Here's how the part is built. I have some questions about the finished solid (model axes, mm). A direction names the side the tool comes from. Round coordinates to 2 decimals unless told otherwise and drop trailing zeros. Loops run counter-clockwise (first coordinate to the right, second up) from the corner with the lowest first, then second, coordinate; pieces in that order, holes last. Notation, with made-up numbers: (35.5, 80) -> (91.5, 80) arc R19 ccw to (91.5, 98) -> close; hole circle Ø8 at (71.25, 54). An arc over 180 degrees is marked (long way). Use one line per item in the form item = value. Start each with the question number.
Item 1: If we section it at C-C (x = 14): Write out the boundary of the cut face in (y, z), then the cut area to 3 significant figures.
Item 2: If I drill on L1, parallel to Y at x = 0.5, z = 3.75 (3 decimals); L2, parallel to X at y = 0, z = 6 (3 decimals); L3, parallel to Y at x = -2, z = 1.25, over which ranges is the centre line in solid material (lowest first)? Write a range as [from, to].
Item 3: For faces 4 (the face through (12.92, -21.56, 4.93)), 5 (the face through (2.865, 20.849, 5.07)), 6 (the face through (-2.15, 18, 5)), 7 (the face through (-3.15, 19, 5)), which set-ups out of +Z, -Z, +X, -X, +Y, -Y let a thin tool reach every point of the face, with its end or its side?
Item 4: Thinking about a two-plate mould opening in X: for faces 1 (the face through (15.558, 3.798, 4.93)), 2 (the face through (-2.15, -23, 5)), 3 (the face through (-10.68, -12.86, 5.07)), which applies, released by +X, released by -X, zero draft, split by the parting line, or undercut?
Item 5: If we section it at D-D (y = 9): Write out the boundary of the cut face in (x, z).
Item 6: I'm going to push flat-ended pins straight in: pin 1 Ø1 at (y, z) = (-11.5, 5) entering from -X; pin 2 Ø1.6 at (y, z) = (19, 6.5) entering from -X; pin 3 Ø1.6 at (y, z) = (-24, 5.5) entering from +X. Where does each tip first touch, or does it pass through?
Item 7: If we section it at A-A (y = 0): Write out the boundary of the cut face in (x, z) (3 decimals), then the cut area to 3 significant figures.
Item 8: If we section it at B-B (x = 0): Write out the boundary of the cut face in (y, z) (3 decimals), then the cut area to 4 significant figures.
Autodesk Inventor part; units mm, degrees
ref_plane "YZ Plane" through (0, 0, 0) normal (1, 0, 0) x (0, 1, 0)
ref_plane "XZ Plane" through (0, 0, 0) normal (0, 1, 0) x (-1, 0, 0)
ref_plane "XY Plane" through (0, 0, 0) normal (0, 0, 1) x (1, 0, 0)
sketch "Sketch1" plane through (0, 0, 0) normal (0, 0, 1) x (1, 0, 0)
  circle A0 centre (0, 0) radius 15.015
  circle A1 centre (0, 0) radius 16.015
  line L0 (-10, -12.5092) -> (-15, -28)
  line L1 (-15, -28) -> (15, -28)
  line L2 (15, -28) -> (10, -12.5092)
  line L3 (8.2846, -13.7057) -> (11.9301, -25)
  line L4 (11.9301, -25) -> (3.15, -25)
  line L5 (-11.9301, -25) -> (-8.2846, -13.7057)
  line L6 (-1.5, -14.9399) -> (-1.5, -14.515)
  line L7 (-1, -14.015) -> (1, -14.015)
  line L8 (1.5, -14.515) -> (1.5, -14.9399)
  arc A2 (-1, -14.015) -> (-1.5, -14.515) centre (-1, -14.515) ccw
  arc A3 (1.5, -14.515) -> (1, -14.015) centre (1, -14.515) ccw
  line L9 (2, -25) -> (2, -22) construction
  line L10 (2, -22) -> (-2, -22) construction
  line L11 (-2, -22) -> (-2, -25) construction
  line L12 (-2.15, -25) -> (-2.15, -21.85)
  line L13 (-2.15, -21.85) -> (2.15, -21.85)
  line L14 (2.15, -21.85) -> (2.15, -25)
  line L15 (-3.15, -25) -> (-3.15, -20.85)
  line L16 (-3.15, -20.85) -> (3.15, -20.85)
  line L17 (3.15, -20.85) -> (3.15, -25)
  line L18 (3.15, -25) -> (2.15, -25)
  line L19 (2.15, -25) -> (-2.15, -25)
  line L20 (-2.15, -25) -> (-3.15, -25)
  line L21 (-3.15, -25) -> (-11.9301, -25)
  line L22 (2, 20) -> (-2, 20) construction
  line L23 (-2, 20) -> (-2, 17) construction
  line L24 (-2, 17) -> (2, 17) construction
  line L25 (2, 17) -> (2, 20) construction
  line L26 (-2.15, 16.85) -> (-2.15, 20.15)
  line L27 (-2.15, 20.15) -> (2.15, 20.15)
  line L28 (2.15, 20.15) -> (2.15, 16.85)
  line L29 (2.15, 16.85) -> (-2.15, 16.85)
  line L30 (3.15, 15.7022) -> (3.15, 21.15)
  line L31 (3.15, 21.15) -> (-3.15, 21.15)
  line L32 (-3.15, 21.15) -> (-3.15, 15.7022)
  point P0 (0, -28)
  point P1 (-1.5, -14.015)
  point P2 (1.5, -14.015)
  point P3 (0, -14.015)
  point P4 (0, -15.015)
  point P5 (0, -22)
  point P6 (0, -25)
  point P7 (0, -25)
  point P8 (0, 17)
  dimension "d0" = 28
  dimension "d1" = 1
  dimension "d2" = 30
  dimension "d3" = 30.03
  dimension "d4" = 20
  dimension "d5" = 3
  dimension "d6" = 2
  dimension "d10" = 3
  dimension "d12" = 1
  dimension "d13" = 0.5
  dimension "d14" = 3
  dimension "d15" = 4
  dimension "d16" = 0.15
  dimension "d17" = 1
  dimension "d21" = 4
  dimension "d22" = 3
  dimension "d23" = 17
  dimension "d24" = 0.15
  dimension "d25" = 1
  dimension "d26" = 1
  dimension "d27" = 1
extrude "Extrusion1" add sketch "Sketch1" along normal blind 10 contours L6 A2 L7 A3 L8 A0 | A1 | A1 L32 L31 L30 | L2 L1 L0 A1 L5 L21 L20 L19 L18 L4 L3 | L18 L14 L13 L12 L20 L15 L16 L17 picked at (0.1669, -14.3455)
fillet "Fillet1" radius 4 6 edges at (10, -12.5092, 5) (8.2846, -13.7057, 5) (-8.2846, -13.7057, 5) (-10, -12.5092, 5) (3.15, 15.7022, 5) (-3.15, 15.7022, 5)
fillet "Fillet1" radius 2 4 edges at (11.9301, -25, 5) (-11.9301, -25, 5) (-3.15, -25, 5) (3.15, -25, 5)
fillet "Fillet1" radius 1 4 edges at (3.15, -20.85, 5) (-3.15, -20.85, 5) (3.15, 21.15, 5) (-3.15, 21.15, 5)
properties part number "Motor Reversed Mount Midsection" material "ABS Plastic"
Values found:
q1.outline = (-28, 0) -> (-24.9, 0) -> (-24.9, 10) -> (-28, 10) -> close; (-7.78, 0) -> (-5.43, 0) -> (-5.43, 10) -> (-7.78, 10) -> close; (5.43, 0) -> (7.78, 0) -> (7.78, 10) -> (5.43, 10) -> close
q1.area = 78.0 mm2
q2.L1 = [-28, -25], [-21.85, -20.85], [-16.007, -14.015], [15.007, 16.85], [20.15, 21.15]
q2.L2 = [-16.015, -15.015], [15.015, 16.015]
q2.L3 = [-28, -25], [-21.85, -20.85], [-15.89, -14.88], [14.88, 16.85], [20.15, 21.15]
q3.face_4 = +Z, -Z, +X
q3.face_5 = +Z, -Z, +X, +Y
q3.face_6 = +Z, -Z
q3.face_7 = +Z, -Z, -X, +Y
q4.face_1 = released by +X
q4.face_2 = undercut
q4.face_3 = released by -X
q5.outline = (-13.25, 0) -> (-12.02, 0) -> (-12.02, 10) -> (-13.25, 10) -> close; (12.02, 0) -> (13.25, 0) -> (13.25, 10) -> (12.02, 10) -> close
q6.pin_1 = -11.64
q6.pin_2 = -3.18
q6.pin_3 = 13.97
q7.outline = (-16.015, 0) -> (-15.015, 0) -> (-15.015, 10) -> (-16.015, 10) -> close; (15.015, 0) -> (16.015, 0) -> (16.015, 10) -> (15.015, 10) -> close
q7.area = 20.0 mm2
q8.outline = (-28, 0) -> (-25, 0) -> (-25, 10) -> (-28, 10) -> close; (-21.85, 0) -> (-20.85, 0) -> (-20.85, 10) -> (-21.85, 10) -> close; (-16.015, 0) -> (-14.015, 0) -> (-14.015, 10) -> (-16.015, 10) -> close; (15.015, 0) -> (16.85, 0) -> (16.85, 10) -> (15.015, 10) -> close; (20.15, 0) -> (21.15, 0) -> (21.15, 10) -> (20.15, 10) -> close
q8.area = 88.35 mm2
